```python
from build123d import *

# Parameters (mm, degrees)
BOSS_EXTRUDE1_DEPTH                          = 28
CSK_FOR_M3_COUNTERSUNK_FLAT_HEAD_SCR_2_COUNT = 2
CSK_FOR_M3_COUNTERSUNK_FLAT_HEAD_SCR_2_PITCH = 13


with BuildPart() as part:
    # Sketch1 → Boss-Extrude1 (new body)
    with BuildSketch(Plane(origin=(0, 0, 0), x_dir=(0, 0, -1), z_dir=(1, 0, 0))):
        Polygon((-10, 0), (0, 0), (0, 15), (-2, 15), (-2, 2), (-10, 2), align=None)
    extrude(amount=BOSS_EXTRUDE1_DEPTH)

    # Sketch3 → CSK for M3 Countersunk Flat Head Screw1 (revolve, cut)
    with BuildSketch(Plane(origin=(7.5, 2, 5.5), x_dir=(0, 0, 1), z_dir=(1, 0, 0))):
        Polygon((0, 0), (0, 2), (1.7, 2), (1.7, 1.45), (3.15, 0), align=None)
    csk_for_m3_countersunk_flat_head_screw1 = revolve(axis=Axis((7.5, 8.35, 5.5), (0, -1, 0)), mode=Mode.SUBTRACT)

    # CSK for M3 Countersunk Flat Head Scr 2: CSK for M3 Countersunk Flat Head Screw1 ×2
    with Locations(*[(i * CSK_FOR_M3_COUNTERSUNK_FLAT_HEAD_SCR_2_PITCH, 0, 0) for i in range(1, CSK_FOR_M3_COUNTERSUNK_FLAT_HEAD_SCR_2_COUNT)]):
        add(csk_for_m3_countersunk_flat_head_screw1, mode=Mode.SUBTRACT)


solid = part.part
```
Verification items for the finished model (mm, model axes). A direction names the side the tool comes from. Give positions to 0.01 mm unless a question says otherwise; leave off trailing zeros. Loops run counter-clockwise (first coordinate to the right, second up) from the corner with the lowest first, then second, coordinate; pieces in that order, holes last. Notation, with made-up numbers: M -24.5,56 L 0.5,56 A10 ccw 0.5,65 Z; hole C -21.5,35 d2. An arc over 180 degrees is marked long. One line per question, with ' | ' between items.
Item 1: Section check B-B, the plane z = 5.5. Record the cut outline in (x, y), plus the area to 3 significant figures.
Completed:
outline: M 0,0 L 5.8,0 L 5.8,0.55 L 4.35,2 L 0,2 Z; M 9.2,0 L 18.8,0 L 18.8,0.55 L 17.35,2 L 10.65,2 L 9.2,0.55 Z; M 22.2,0 L 28,0 L 28,2 L 23.65,2 L 22.2,0.55 Z | area: 38.2 mm^2
Item 2: Depth check by flat-ended pin: P1, Ø2, axis at x = 19, y = 13.5, coming from the +Z side; P2, Ø5, axis at x = 5, z = 8, coming from the +Y side. Enter the tip coordinate at first touch or a pass-through.
Completed:
P1: stops at z = 2 | P2: stops at y = 2
Item 3: Section check C-C, the plane x = 3.75. Record the cut outline in (y, z), plus the area to 3 significant figures.
Completed:
outline: M 0,0 L 15,0 L 15,2 L 2,2 L 2,10 L 0,10 Z | area: 46.0 mm^2
Item 4: Draft check along Z on faces 3 (the face through (9.16, 0.28, 5.13)), 4 (the face through (14, 7, 0)), 5 (the face through (14, 0, 5)), 6 (the face through (14, 9, 2)). Enter one of: +Z half, -Z half, draft (parallel to the pull), parting line (faces both ways), or undercut.
Completed:
face 3: undercut | face 4: -Z half | face 5: draft | face 6: +Z half
Item 5: Tool access check on faces 1 (the face through (14, 2, 6)), 2 (the face through (0, 5.3, 1.7)). Record the directions out of +Z, -Z, +X, -X, +Y, -Y that give a thin tool (end or side, any length) a straight path to the whole face; none if there is none.
Completed:
face 1: +Z, +X, -X, +Y | face 2: +Z, -Z, -X, +Y, -Y
Item 6: Thickness scan on line 1 (X direction, y = 0.2, z = 5.5); line 2 (Z direction, x = 7.5, y = 0.3); line 3 (Y direction, x = 25.25, z = 6). Record the ranges inside material, lowest first. Write a range as [from, to].
Completed:
line 1: x = [0, 5.8], [9.2, 18.8], [22.2, 28] | line 2: z = [0, 3.8], [7.2, 10] | line 3: y = [0, 2]
Item 7: Section check D-D, the plane y = 11.25. Record the cut outline in (x, z), plus the area to 3 significant figures.
Completed:
outline: M 0,0 L 28,0 L 28,2 L 0,2 Z | area: 56.0 mm^2
Item 8: Section check A-A, the plane x = 7.5. Record the cut outline in (y, z).
Completed:
outline: M 0,0 L 15,0 L 15,2 L 2,2 L 2,2.35 L 0.55,3.8 L 0,3.8 Z; M 0,7.2 L 0.55,7.2 L 2,8.65 L 2,10 L 0,10 Z
